```python
from build123d import *

# Parameters (mm, degrees)
SKETCH1_R               = 8
BOSS_EXTRUDE1_DEPTH     = 7
SKETCH2_R               = 5
BOSS_EXTRUDE2_DEPTH     = 10
CUT_EXTRUDE1_DEPTH      = 10
CUT_EXTRUDE1_DEPTH_BACK = 10
SKETCH3_W               = 4
SKETCH3_H               = 4
SKETCH4_R               = 4
BOSS_EXTRUDE3_DEPTH     = 12


with BuildPart() as part:
    # Sketch1 → Boss-Extrude1 (new body)
    with BuildSketch(Plane(origin=(0, 0, 0), x_dir=(1, 0, 0), z_dir=(0, 1, 0))):
        with Locations(Location((0, 0, 0), (0, 0, 270))):
            Circle(SKETCH1_R)
    extrude(amount=-BOSS_EXTRUDE1_DEPTH)

    # Sketch2 → Boss-Extrude2 (add)
    with BuildSketch(Plane(origin=(0, 0, 0), x_dir=(1, 0, 0), z_dir=(0, 1, 0))):
        with Locations(Location((0, 0, 0), (0, 0, 270))):
            Circle(SKETCH2_R)
    extrude(amount=BOSS_EXTRUDE2_DEPTH)

    # Sketch3 → Cut-Extrude1 (cut, two sides: drawn at the far end of the back side and taken through both)
    with BuildSketch(Plane(origin=(0, 0, 0), x_dir=(0, 0, -1), z_dir=(1, 0, 0)).offset(-CUT_EXTRUDE1_DEPTH_BACK)):
        with Locations((0, -5)):
            Rectangle(SKETCH3_W, SKETCH3_H)
    extrude(amount=CUT_EXTRUDE1_DEPTH + CUT_EXTRUDE1_DEPTH_BACK, mode=Mode.SUBTRACT)

    # Sketch4 → Boss-Extrude3 (add)
    with BuildSketch(Plane(origin=(0, 10, 0), x_dir=(1, 0, 0), z_dir=(0, 1, 0))):
        with Locations(Location((0, 0, 0), (0, 0, 270))):
            Circle(SKETCH4_R)
    extrude(amount=BOSS_EXTRUDE3_DEPTH)


solid = part.part
```
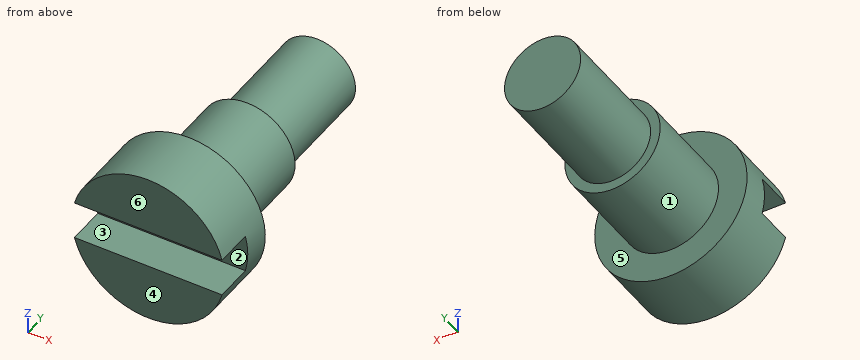
For this review, take the finished solid that the model builds, in its own axes (mm). Face numbers are marked on the shaded views. A direction names the side the tool comes from. Round coordinates to 2 decimals unless told otherwise and drop trailing zeros. Write each loop counter-clockwise with the first axis right and the second up, starting at its lowest first coordinate (ties: lowest second). Pieces come first, ordered by that corner, then holes. Notation, with made-up numbers: M 47.25,53.5 L 97.25,53.5 A10 cw 97.25,66.5 Z; hole C 21.5,-35.75 d10. An arc over 180 degrees is marked long. One line per item, written item: value. Start each with the question number.
(1) We need section A-A (z = 0). Give the boundary of the cut face in (x, y), and give its area (3 significant figures).
(2) The part is to be moulded in two halves that separate along Z. For the marked faces 1, 2, 3 and 4, say which applies: released by +Z, released by -Z, zero draft, split by the parting line, or undercut.
(3) Insertion check: pin 1 (3 mm diameter, centred on x = -5.5, y = -4, fed in from +Z); pin 2 (2 mm diameter, centred on x = -1, z = 0.5, fed in from -Y); pin 3 (6 mm diameter, centred on y = 16.5, z = 0.5, fed in from -X). Each pin has a flat end and moves straight along its axis. Give the tip position at first contact, or say it passes through.
(4) We need section D-D (x = -6.5). Give the boundary of the cut face in (y, z), and give its area (3 significant figures).
(5) We need section C-C (y = -0.75). Give the boundary of the cut face in (x, z), and give its area (3 significant figures).
(6) Machinability: for the marked faces 5 and 6, which of the approach directions +Z, -Z, +X, -X, +Y, -Y give a long, thin tool a straight path to every point of the face, cutting with its end or side? Answer none if there is none.
(7) Wall thickness on line 1 (Y direction, x = 4.5, z = 0.25); line 2 (Y direction, x = 1.5, z = -0.75); line 3 (Z direction, x = -3, y = -5.5): over which ranges is each line inside the solid? List them lowest first.
(8) We need section B-B (x = 0). Give the boundary of the cut face in (y, z), and give its area (3 significant figures).
Result:
1. outline: M -8,-3 L 8,-3 L 8,0 L 5,0 L 5,10 L 4,10 L 4,22 L -4,22 L -4,10 L -5,10 L -5,0 L -8,0 Z
1. area: 244 mm²
2. face 1: split by the parting line
2. face 2: undercut
2. face 3: undercut
2. face 4: zero draft
3. pin 1: z = 6.93
3. pin 2: y = -3
3. pin 3: x = -4
4. outline: M -7,-4.66 L 0,-4.66 L 0,4.66 L -7,4.66 L -7,2 L -3,2 L -3,-2 L -7,-2 Z
4. area: 49.3 mm²
5. outline: C 0,0 d16
5. area: 201 mm²
6. face 5: +Y
6. face 6: +Z, -Z, +X, -X, -Y
7. line 1: -3 to 10
7. line 2: -3 to 22
7. line 3: -7.42 to -2, 2 to 7.42
8. outline: M -7,-8 L 0,-8 L 0,-5 L 10,-5 L 10,-4 L 22,-4 L 22,4 L 10,4 L 10,5 L 0,5 L 0,8 L -7,8 L -7,2 L -3,2 L -3,-2 L -7,-2 Z
8. area: 292 mm²
